The figure shows three views and two pictorial views of one solid part (mm, origin at its lowest corner). Answer the questions. A direction names the side the tool comes from. Give positions to 0.01 mm unless a question says otherwise; leave off trailing zeros. Order: outer loops, then holes, each group sorted by start corner. A loop starts at its lowest first (then second) coordinate and runs counter-clockwise, first axis right, second up. Notation, with made-up numbers: M -11.5,43 L 26.5,43 A24 cw 26.5,59 Z; hole C -7.75,49 d2. An arc over 180 degrees is marked long. Write item = value, one per line. Start each with the question number.
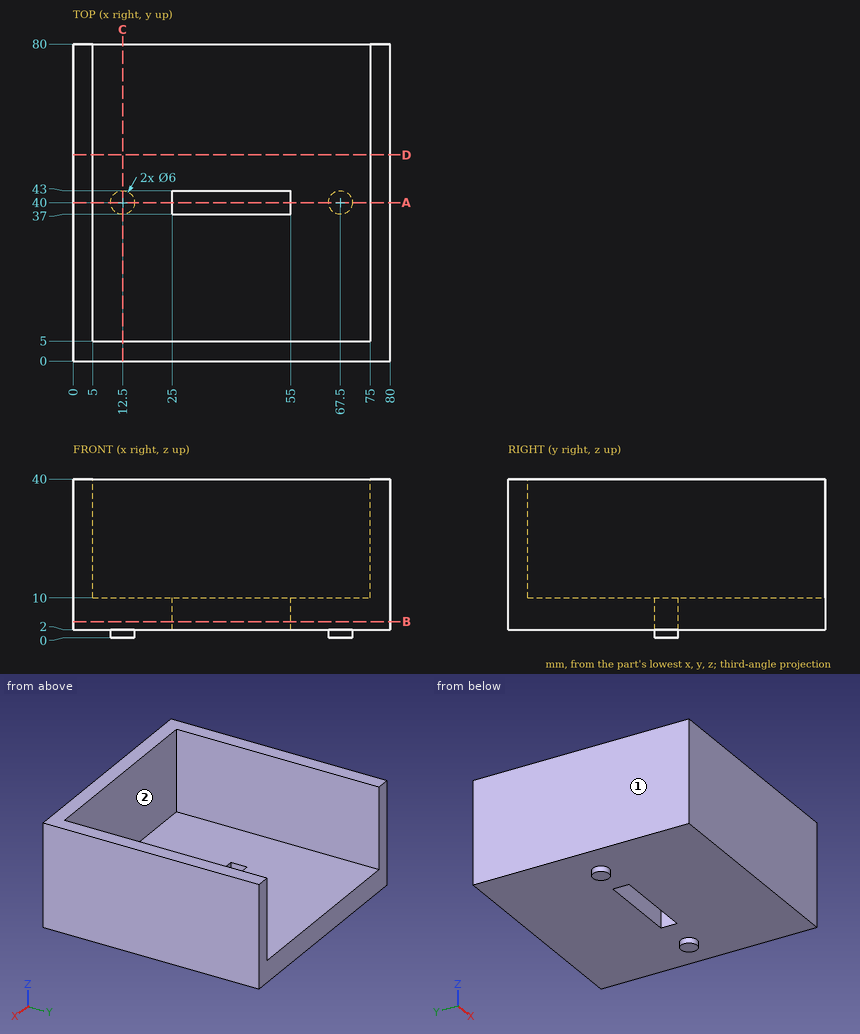
1) Find section C-C on x = 12.5. Determine the outline of the cut face in (y, z), plus the area to 3 significant figures.
2) Find the intervals of material crossed by probe 1 along X at (y, z) = (26, 35); probe 2 along Y at (x, z) = (41.5, 28); probe 3 along Z at (x, y) = (5.5, 12), in increasing order. Write a range as [from, to].
3) Find section D-D on y = 52. Determine the outline of the cut face in (x, z), plus the area to 3 significant figures.
4) For the marked faces 1 and 2, determine the directions among +Z, -Z, +X, -X, +Y, -Y from which every point of the face is accessible in a straight line to the end or side of a thin tool.
5) Find section A-A on y = 40. Determine the outline of the cut face in (x, z).
6) Find section B-B on z = 4. Determine the outline of the cut face in (x, y).
7) Each of these flat-tipped pins is pushed along its axis until it touches: P1, Ø6.5, axis at x = 43.5, z = 5, coming from the -Y side; P2, Ø1, axis at x = 24, y = 51, coming from the -Z side; P3, Ø5, axis at x = 67, y = 16.5, coming from the +Z side; P4, Ø9, axis at x = 41.5, z = 30, coming from the +Y side. Where does it stop, or does it pass through?
Numbers:
q1.outline = M 0,2 L 37,2 L 37,0 L 43,0 L 43,2 L 80,2 L 80,10 L 5,10 L 5,40 L 0,40 Z
q1.area = 802 mm2
q2.probe_1 = [0, 5], [75, 80]
q2.probe_2 = [0, 5]
q2.probe_3 = [2, 10]
q3.outline = M 0,2 L 80,2 L 80,40 L 75,40 L 75,10 L 5,10 L 5,40 L 0,40 Z
q3.area = 940 mm2
q4.face_1 = +Z, -Z, -X, +Y, -Y
q4.face_2 = +Z, +Y
q5.outline = M 0,2 L 9.5,2 L 9.5,0 L 15.5,0 L 15.5,2 L 25,2 L 25,10 L 5,10 L 5,40 L 0,40 Z; M 55,2 L 64.5,2 L 64.5,0 L 70.5,0 L 70.5,2 L 80,2 L 80,40 L 75,40 L 75,10 L 55,10 Z
q6.outline = M 0,0 L 80,0 L 80,80 L 0,80 Z; hole M 25,37 L 55,37 L 55,43 L 25,43 Z
q7.P1 = 0
q7.P2 = 2
q7.P3 = 10
q7.P4 = 5
